from build123d import *

# Parameters (mm, degrees)
F0_W     = 70
F0_H     = 100
F1_DEPTH = 7
F2_R     = 2
F3_R     = 1.25
F3_W     = 44.0106242895
F3_H     = 4.7012990341
F4_DEPTH = 3


with BuildPart() as f1:
    # F0 (on Front) → F1 (new body)
    with BuildSketch(Plane.XZ):
        with Locations((43.885584152, 59.9958246574)):
            Rectangle(F0_W, F0_H)
    extrude(amount=F1_DEPTH)

    # F2
    f2_edges = [f1.edges().sort_by_distance(p)[0] for p in [
        (8.885584, -3.5, 109.995825),
        (8.885584, -3.5, 9.995825),
        (78.885584, -3.5, 9.995825),
        (78.885584, -3.5, 109.995825),
    ]]
    fillet(f2_edges, radius=F2_R)

    # F3 (on face) → F4 (cut)
    with BuildSketch(Plane.XZ.offset(7)):
        with Locations((13.025584152, 95.9958246574)):
            Circle(F3_R)
        with Locations((74.745584152, 95.9958246574)):
            Circle(F3_R)
        with Locations((13.025584152, 19.3958246574)):
            Circle(F3_R)
        with Locations((74.745584152, 19.3958246574)):
            Circle(F3_R)
        with Locations((39.9450175464, 107.6451751404)):
            Rectangle(F3_W, F3_H)
    extrude(amount=-F4_DEPTH, mode=Mode.SUBTRACT)


solid = f1.part
Read the model definition and answer for the solid it produces. Units are mm, in the model's axes. A direction names the side the tool comes from. Round coordinates to 2 decimals unless told otherwise and drop trailing zeros. Write each loop counter-clockwise with the first axis right and the second up, starting at its lowest first coordinate (ties: lowest second). Pieces come first, ordered by that corner, then holes.
Q1. Find section A-A on x = 19. Determine the outline of the cut face in (y, z), and give its area (3 significant figures).
Values:
outline: (-7, 10) - (0, 10) - (0, 110) - (-4, 110) - (-4, 105.29) - (-7, 105.29) - close
area: 686 mm2
Q2. The mould has two halves that part along X. Classify faces 4 (the face through (40, -4, 108)), 5 (the face through (78.284, -3.549, 10.566)), 6 (the face through (43, 0, 61)): released by +X, released by -X, zero draft, split by the parting line, or undercut.
Values:
face 4: undercut
face 5: released by +X
face 6: zero draft
Q3. Find section B-B on y = -6. Determine the outline of the cut face in (x, z).
Values:
outline: (8.89, 12) arc R2 ccw to (10.89, 10) - (76.89, 10) arc R2 ccw to (78.89, 12) - (78.89, 108) arc R2 ccw to (76.89, 110) - (61.95, 110) - (61.95, 105.29) - (17.94, 105.29) - (17.94, 110) - (10.89, 110) arc R2 ccw to (8.89, 108) - close; hole circle Ø2.5 at (13.03, 19.4); hole circle Ø2.5 at (13.03, 96); hole circle Ø2.5 at (74.75, 19.4); hole circle Ø2.5 at (74.75, 96)
Q4. Straight lines are drawn through the part: line 1 (Z direction, x = 50, y = -6.5); line 2 (X direction, y = -5.5, z = 19). For each, find the intervals that lie inside material, in ascending order.
Values:
line 1: z = 10 to 105.29
line 2: x = 8.89 to 11.84, 14.21 to 73.56, 75.93 to 78.89
Q5. Flat-ended cylindrical pins translate along their axes: P1, Ø1.2, axis at x = 74.5, z = 95.5, coming from the -Y side; P2, Ø3.5, axis at x = 49.5, y = -6, coming from the +Z side. Find the tip coordinate at first contact, or state that the pin passes through.
Values:
P1: stops at y = -4
P2: stops at z = 105.29
Q6. A tool of negligible diameter and unlimited length cuts with its end or side. For faces 1 (the face through (43, -7, 61)), 2 (the face through (40, -6, 105.295)), 3 (the face through (75.94, -5.52, 96.37)), from which of +Z, -Z, +X, -X, +Y, -Y can it reach the whole face along a straight path? Write none if from no direction.
Values:
face 1: +Z, -Z, +X, -X, -Y
face 2: +Z, -Y
face 3: -Y
